CAD build for the part. Positions are in the model's coordinates, mm. Face numbers are marked on the shaded views. Give positions to 0.01 mm unless a question says otherwise; leave off trailing zeros. Loops run counter-clockwise (first coordinate to the right, second up) from the corner with the lowest first, then second, coordinate; pieces in that order, holes last. Notation, with made-up numbers: (-17.5, 61.25) - (-8.5, 61.25) arc R22 cw to (-8.5, 87.25) - close; hole circle Ø1 at (24, -20.75). An arc over 180 degrees is marked (long way). Return JSON: item names as keys, results as strings.
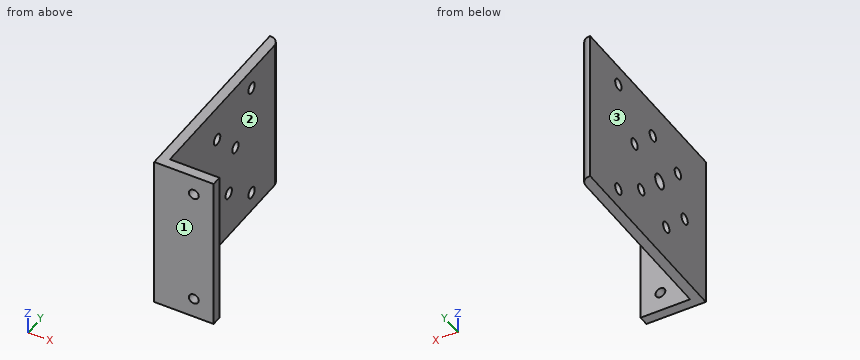
from build123d import *

# Parameters (mm, degrees)
BOSS_EXTRUDE1_DEPTH     = 100.4
SKETCH2_R               = 4.7625
SKETCH2_R_2             = 3.5
CUT_EXTRUDE1_DEPTH      = 1
CUT_EXTRUDE1_DEPTH_BACK = 39.1
SKETCH3_R               = 3.175
CUT_EXTRUDE2_DEPTH      = 7.35
SKETCH5_R               = 3.5
CUT_EXTRUDE4_DEPTH      = 10


with BuildPart() as part:
    # Sketch1 → Boss-Extrude1 (new body)
    with BuildSketch(Plane.XY):
        with BuildLine():
            Line((0, 6.35), (0, 0))
            Line((0, 0), (38.1, 0))
            Line((38.1, 0), (38.1, 0.35))
            Line((38.1, 0.35), (38.1, 6.35))
            Line((38.1, 6.35), (32.1, 6.35))
            Line((32.1, 6.35), (6.35, 6.35))
            Line((6.35, 6.35), (6.35, 37.75))
            Line((6.35, 37.75), (6.35, 121))
            ThreePointArc((6.35, 121), (4.592640687, 125.242640687), (0.35, 127))
            Line((0.35, 127), (0, 127))
            Line((0, 127), (0, 6.35))
        make_face()
    extrude(amount=BOSS_EXTRUDE1_DEPTH)

    # Sketch2 → Cut-Extrude1 (cut, two sides)
    with BuildSketch(Plane.ZY) as cut_extrude1_sk:
        with Locations((50.2, 50.8)):
            Circle(SKETCH2_R)
        with Locations((57.576342785, 78.328886049)):
            Circle(SKETCH2_R_2)
        with Locations((30.047456736, 70.952543264)):
            Circle(SKETCH2_R_2)
        with Locations((22.671113951, 43.423657215)):
            Circle(SKETCH2_R_2)
        with Locations((42.823657215, 23.271113951)):
            Circle(SKETCH2_R_2)
        with Locations((70.352543264, 30.647456736)):
            Circle(SKETCH2_R_2)
        with Locations((77.728886049, 58.176342785)):
            Circle(SKETCH2_R_2)
    extrude(amount=CUT_EXTRUDE1_DEPTH, mode=Mode.SUBTRACT)
    extrude(cut_extrude1_sk.sketch, amount=-CUT_EXTRUDE1_DEPTH_BACK, mode=Mode.SUBTRACT)

    # Sketch3 → Cut-Extrude2 (cut, through all)
    with BuildSketch(Plane(origin=(0, 6.35, 0), x_dir=(1, 0, 0), z_dir=(0, 1, 0))):
        with Locations((25.4, -12.7)):
            Circle(SKETCH3_R)
        with Locations((25.4, -87.7)):
            Circle(SKETCH3_R)
    extrude(amount=-CUT_EXTRUDE2_DEPTH, mode=Mode.SUBTRACT)

    # Sketch5 → Cut-Extrude4 (cut)
    with BuildSketch(Plane(origin=(6.35, 0, 0), x_dir=(0, 0, -1), z_dir=(1, 0, 0))):
        with Locations((-87.7, 96)):
            Circle(SKETCH5_R)
        with Locations((-12.7, 96)):
            Circle(SKETCH5_R)
    extrude(amount=-CUT_EXTRUDE4_DEPTH, mode=Mode.SUBTRACT)


solid = part.part
1. Cut at D-D, the plane z = 64.5. Write the cut outline in (x, y).
Values follow:
{"outline": "(0, 0) - (38.1, 0) - (38.1, 6.35) - (6.35, 6.35) - (6.35, 121) arc R6 ccw to (0.35, 127) - (0, 127) - close"}
2. Cut at C-C, the plane y = 50.8. Write the cut outline in (x, z).
Values follow:
{"outline": "(0, 0) - (6.35, 0) - (6.35, 45.44) - (0, 45.44) - close; (0, 54.96) - (6.35, 54.96) - (6.35, 100.4) - (0, 100.4) - close"}
3. Cut at A-A, the plane x = 25.4. Write the cut outline in (y, z) (3 decimals).
Values follow:
{"outline": "(0, 0) - (6.35, 0) - (6.35, 9.525) - (0, 9.525) - close; (0, 15.875) - (6.35, 15.875) - (6.35, 84.525) - (0, 84.525) - close; (0, 90.875) - (6.35, 90.875) - (6.35, 100.4) - (0, 100.4) - close"}
4. Drop flat-ended pins along their axis: P1, Ø10, axis at x = 12, z = 79.5, coming from the -Y side; P2, Ø6.5, axis at y = 96, z = 12.7, coming from the -X side; P3, Ø1, axis at x = 32, z = 53, coming from the +Y side; P4, Ø5, axis at y = 67, z = 77, coming from the +X side. Give the stop position or say it passes through.
Values follow:
{"P1": "stops at y = 0", "P2": "passes through", "P3": "stops at y = 6.35", "P4": "stops at x = 6.35"}
5. Cut at B-B, the plane z = 87.7. Write the cut outline in (x, y) (3 decimals), plus the area to 3 significant figures.
Values follow:
{"outline": "(0, 0) - (22.225, 0) - (22.225, 6.35) - (6.35, 6.35) - (6.35, 92.5) - (0, 92.5) - close; (0, 99.5) - (6.35, 99.5) - (6.35, 121) arc R6 ccw to (0.35, 127) - (0, 127) - close; (28.575, 0) - (38.1, 0) - (38.1, 6.35) - (28.575, 6.35) - close", "area": "916 mm²"}
6. Pull direction X, two halves, no side cores. Call the marked faces 1, 2 and 3: +X half, -X half, draft (parallel to the pull), parting line (faces both ways), or undercut.
Values follow:
{"face 1": "draft", "face 2": "+X half", "face 3": "-X half"}
7. Drill centre lines: probe 1 along Z at (x, y) = (25.4, 2) (3 decimals); probe 2 along Z at (x, y) = (5, 70.5); probe 3 along Y at (x, z) = (23, 63.5). Where is each one in solid material? Low to high.
Values follow:
{"probe 1": "z = 0 to 9.525, 15.875 to 84.525, 90.875 to 100.4", "probe 2": "z = 0 to 26.58, 33.52 to 100.4", "probe 3": "y = 0 to 6.35"}
